For this review, use the dimensioned drawing (mm, ordinates from the lowest corner) and the shaded views. A direction names the side the tool comes from. Round coordinates to 2 decimals unless told otherwise and drop trailing zeros. Order: outer loops, then holes, each group sorted by start corner. A loop starts at its lowest first (then second) coordinate and runs counter-clockwise, first axis right, second up. Notation, with made-up numbers: (14, 55) -> (34, 55) arc R17 cw to (34, 59) -> close; hole circle Ø8 at (-19, 43). An arc over 180 degrees is marked (long way). Answer in a Markdown table with one row per item.
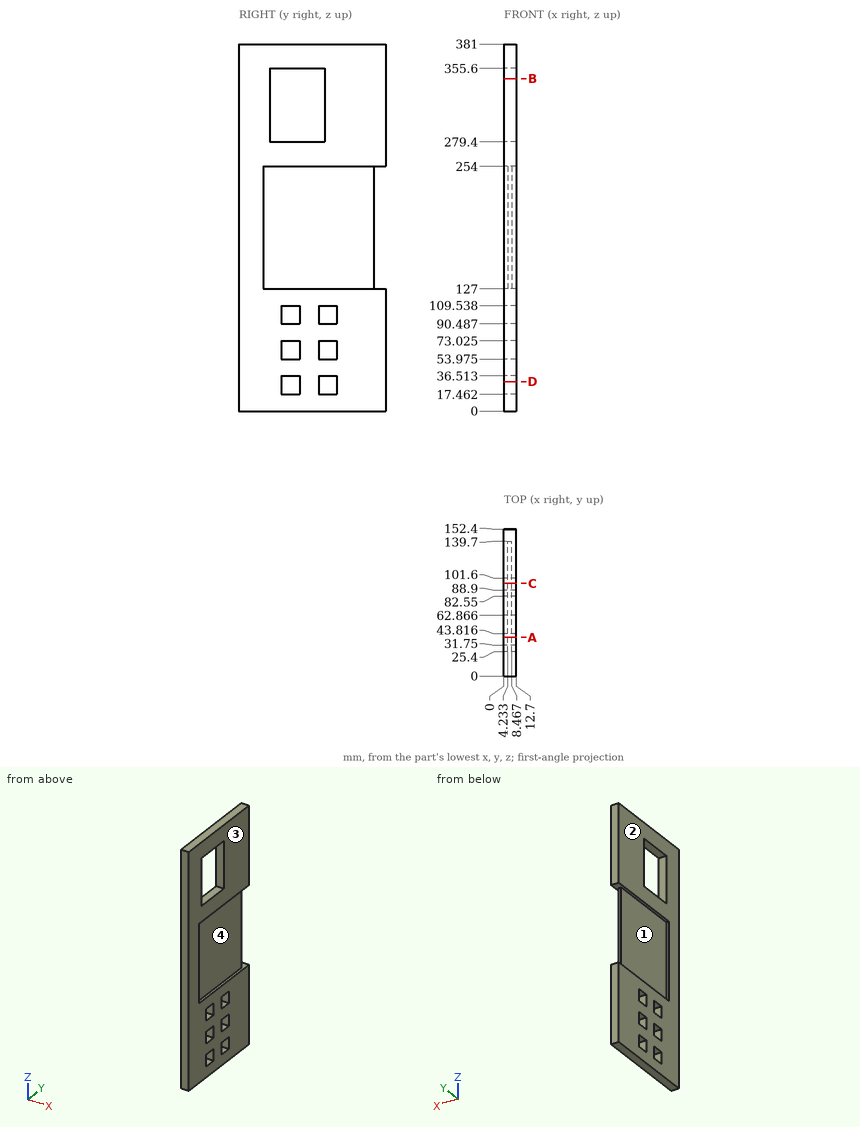
Q1. Take a section at C-C, the plane y = 96. Write out the cut boundary in (x, z) (1 decimal), then the cut area to 3 significant figures.
Answer key:
| item | result |
|---|---|
| outline | (0, 0) -> (12.7, 0) -> (12.7, 17.5) -> (0, 17.5) -> close; (0, 36.5) -> (12.7, 36.5) -> (12.7, 54) -> (0, 54) -> close; (0, 73) -> (12.7, 73) -> (12.7, 90.5) -> (0, 90.5) -> close; (0, 109.5) -> (12.7, 109.5) -> (12.7, 127) -> (8.5, 127) -> (8.5, 254) -> (12.7, 254) -> (12.7, 381) -> (0, 381) -> (0, 254) -> (4.2, 254) -> (4.2, 127) -> (0, 127) -> close |
| area | 3,040 mm^2 |
Q2. To check wall thickness, follow probe 1 along Z at (x, y) = (12, 42); probe 2 along Z at (x, y) = (3.75, 52) (1 decimal); probe 3 along Z at (x, y) = (8.5, 96) (1 decimal). State the ranges of each line that lie inside material, in increasing order.
Answer key:
| item | result |
|---|---|
| probe 1 | z = 0 to 127, 254 to 279.4, 355.6 to 381 |
| probe 2 | z = 0 to 17.5, 36.5 to 54, 73 to 90.5, 109.5 to 127, 254 to 279.4, 355.6 to 381 |
| probe 3 | z = 0 to 17.5, 36.5 to 54, 73 to 90.5, 109.5 to 127, 254 to 381 |
Q3. Clearance check with flat-ended pins moving along their axes: pin 1 Ø2 at (x, z) = (10, 168.5) entering from +Y; pin 2 Ø4.5 at (x, z) = (6, 192) entering from +Y; pin 3 Ø6 at (y, z) = (92, 210.5) entering from -X. State where each tip first meets the part, or that it passes through.
Answer key:
| item | result |
|---|---|
| pin 1 | stops at y = 25.4 |
| pin 2 | stops at y = 139.7 |
| pin 3 | stops at x = 4.23 |
Q4. Take a section at B-B, the plane z = 345. Write out the cut boundary in (x, y).
Answer key:
| item | result |
|---|---|
| outline | (0, 0) -> (12.7, 0) -> (12.7, 31.75) -> (0, 31.75) -> close; (0, 88.9) -> (12.7, 88.9) -> (12.7, 152.4) -> (0, 152.4) -> close |
Q5. Take a section at A-A, the plane y = 40. Write out the cut boundary in (x, z), then the cut area to 3 significant figures.
Answer key:
| item | result |
|---|---|
| outline | (0, 0) -> (12.7, 0) -> (12.7, 127) -> (8.47, 127) -> (8.47, 254) -> (12.7, 254) -> (12.7, 279.4) -> (0, 279.4) -> (0, 254) -> (4.23, 254) -> (4.23, 127) -> (0, 127) -> close; (0, 355.6) -> (12.7, 355.6) -> (12.7, 381) -> (0, 381) -> close |
| area | 2,800 mm^2 |
Q6. The part is to be moulded in two halves that separate along Z. For the marked faces 3 and 4, say which applies: +Z half, -Z half, draft (parallel to the pull), parting line (faces both ways), or undercut.
Answer key:
| item | result |
|---|---|
| face 3 | draft |
| face 4 | undercut |
Q7. Take a section at D-D, the plane z = 30.5. Give the number of separate pieces and of enclosed holes in the cut face, then the cut area to 3 significant figures.
Answer key:
| item | result |
|---|---|
| separate pieces | 3 |
| enclosed holes | 0 |
| area | 1,450 mm^2 |
Q8. Tool access review of the marked faces 1 and 2: name each direction out of +Z, -Z, +X, -X, +Y, -Y from which nothing blocks a thin tool from reaching the whole face with its end or side.
Answer key:
| item | result |
|---|---|
| face 1 | -X, +Y |
| face 2 | +Z, -Z, -X, +Y, -Y |
